```python
from build123d import *

# Parameters (mm, degrees)
F1_DEPTH = 50.8


with BuildPart() as f1:
    # F0 (on Front) → F1 (new body)
    with BuildSketch(Plane.XZ):
        with BuildLine():
            ThreePointArc((22.439383, 29.13105), (15.63549, 24.408793), (9.478033, 18.869985))
            Line((9.478033, 18.869985), (-23.461929, 58.559932))
            ThreePointArc((-23.461929, 58.559932), (-17.627724, 61.636811), (-12.409047, 57.603136))
            ThreePointArc((-12.409047, 57.603136), (-10.811238, 63.430969), (-12.409047, 69.258802))
            ThreePointArc((-12.409047, 69.258802), (-15.886595, 72.352499), (-20.328924, 73.741749))
            ThreePointArc((-20.328924, 73.741749), (-25.439806, 72.849507), (-30.041976, 70.454255))
            ThreePointArc((-30.041976, 70.454255), (-35.3729, 73.298377), (-41.398779, 73.741749))
            ThreePointArc((-41.398779, 73.741749), (-46.195621, 71.631394), (-49.169224, 67.316189))
            ThreePointArc((-49.169224, 67.316189), (-49.483254, 62.267433), (-47.525477, 57.603136))
            ThreePointArc((-47.525477, 57.603136), (-42.391887, 61.189751), (-37.258297, 57.603136))
            Line((-37.258297, 57.603136), (-37.258297, 32.199763))
            ThreePointArc((-37.258297, 32.199763), (-42.167966, 30.518016), (-46.330024, 27.41795))
            ThreePointArc((-46.330024, 27.41795), (-50.063504, 20.954714), (-50.81061, 13.528131))
            ThreePointArc((-50.81061, 13.528131), (-46.942892, 6.36599), (-39.005515, 4.562234))
            ThreePointArc((-39.005515, 4.562234), (-41.07612, 11.736213), (-37.258297, 18.153191))
            Line((-37.258297, 18.153191), (-37.258297, -18.857189))
            ThreePointArc((-37.258297, -18.857189), (-39.487397, -20.916304), (-42.500529, -21.276681))
            ThreePointArc((-42.500529, -21.276681), (-45.274392, -20.531283), (-47.608346, -18.857189))
            ThreePointArc((-47.608346, -18.857189), (-49.230344, -21.155103), (-49.355764, -23.965007))
            ThreePointArc((-49.355764, -23.965007), (-48.428049, -27.320039), (-46.398599, -30.148152))
            ThreePointArc((-46.398599, -30.148152), (-42.216094, -32.810312), (-37.258297, -32.836478))
            ThreePointArc((-37.258297, -32.836478), (-33.318107, -32.162609), (-29.865403, -30.148152))
            ThreePointArc((-29.865403, -30.148152), (-27.712308, -31.840895), (-25.160836, -32.836478))
            ThreePointArc((-25.160836, -32.836478), (-20.455986, -33.443738), (-16.020531, -31.761147))
            ThreePointArc((-16.020531, -31.761147), (-12.932619, -29.265174), (-10.912713, -25.846833))
            ThreePointArc((-10.912713, -25.846833), (-11.2086, -21.67018), (-13.063374, -17.916275))
            ThreePointArc((-13.063374, -17.916275), (-18.372816, -21.371176), (-23.682257, -17.916275))
            Line((-23.682257, -17.916275), (-23.682257, 15.553372))
            ThreePointArc((-23.682257, 15.553372), (-12.957597, 4.154356), (-6.669553, -10.177998))
            Line((-6.669553, -10.177998), (-6.669553, -54.607033))
            ThreePointArc((-6.669553, -54.607033), (-8.287699, -58.119332), (-11.300034, -60.544301))
            ThreePointArc((-11.300034, -60.544301), (-14.772838, -61.47915), (-17.679371, -59.361041))
            ThreePointArc((-17.679371, -59.361041), (-19.114876, -61.809201), (-19.297592, -64.641298))
            ThreePointArc((-19.297592, -64.641298), (-18.536614, -67.512258), (-16.814196, -69.931922))
            ThreePointArc((-16.814196, -69.931922), (-13.12521, -72.407987), (-8.715694, -72.95177))
            ThreePointArc((-8.715694, -72.95177), (-4.221828, -71.834414), (0, -69.931922))
            ThreePointArc((0, -69.931922), (4.559252, -71.907947), (9.41743, -72.95177))
            ThreePointArc((9.41743, -72.95177), (14.035159, -71.901137), (17.746311, -68.959267))
            ThreePointArc((17.746311, -68.959267), (19.072395, -63.743091), (17.746311, -58.526916))
            ThreePointArc((17.746311, -58.526916), (12.125868, -60.902929), (7.176861, -57.333316))
            ThreePointArc((7.176861, -57.333316), (6.708307, -55.925452), (6.564894, -54.448612))
            Line((6.564894, -54.448612), (7.254593, -9.766534))
            ThreePointArc((7.254593, -9.766534), (7.915044, -5.648664), (9.714889, -1.886536))
            Line((9.714889, -1.886536), (22.694213, -18.315103))
            ThreePointArc((22.694213, -18.315103), (17.190391, -21.190166), (11.686569, -18.315103))
            ThreePointArc((11.686569, -18.315103), (10.214197, -22.212635), (10.536366, -26.36653))
            ThreePointArc((10.536366, -26.36653), (13.072681, -30.734713), (17.444285, -33.265127))
            ThreePointArc((17.444285, -33.265127), (23.869566, -32.903906), (29.75891, -30.309618))
            ThreePointArc((29.75891, -30.309618), (35.644058, -32.921994), (42.081258, -32.773871))
            ThreePointArc((42.081258, -32.773871), (45.511296, -30.776469), (47.995683, -27.680892))
            ThreePointArc((47.995683, -27.680892), (48.784561, -22.594925), (46.756167, -17.864702))
            ThreePointArc((46.756167, -17.864702), (41.584109, -21.216198), (36.41205, -17.864702))
            Line((36.41205, -17.864702), (36.41205, 18.417337))
            ThreePointArc((36.41205, 18.417337), (41.00077, 11.851308), (39.371705, 4.008144))
            ThreePointArc((39.371705, 4.008144), (44.606315, 5.931777), (48.501298, 9.923093))
            ThreePointArc((48.501298, 9.923093), (50.482427, 16.674256), (48.501298, 23.425419))
            ThreePointArc((48.501298, 23.425419), (43.576958, 29.192803), (36.828664, 32.652915))
            Line((36.828664, 32.652915), (36.828664, 58.368564))
            ThreePointArc((36.828664, 58.368564), (41.780885, 61.482849), (46.733106, 58.368564))
            ThreePointArc((46.733106, 58.368564), (47.54337, 67.461962), (40.576808, 73.362254))
            ThreePointArc((40.576808, 73.362254), (34.734779, 72.917336), (29.45341, 70.380725))
            ThreePointArc((29.45341, 70.380725), (24.129346, 72.98331), (18.215336, 73.362254))
            ThreePointArc((18.215336, 73.362254), (11.281464, 67.4316), (12.336258, 58.368564))
            ThreePointArc((12.336258, 58.368564), (17.676832, 61.210114), (22.439383, 57.479933))
            Line((22.439383, 57.479933), (22.439383, 29.13105))
        make_face()
        with BuildLine():
            Line((-23.548043, 29.330348), (-23.548043, 39.393221))
            Line((-23.548043, 39.393221), (2.61824, 7.316703))
            Line((2.61824, 7.316703), (0, 1.270827))
            ThreePointArc((0, 1.270827), (-9.020803, 17.611136), (-23.548043, 29.330348))
        make_face(mode=Mode.SUBTRACT)
        with BuildLine():
            ThreePointArc((16.760936, 9.333754), (19.47767, 12.721904), (22.865819, 15.43864))
            Line((22.865819, 15.43864), (22.865819, 1.898702))
            Line((22.865819, 1.898702), (16.760936, 9.333754))
        make_face(mode=Mode.SUBTRACT)
    extrude(amount=F1_DEPTH)


solid = f1.part
```
CAD build for the part. Positions are in the model's coordinates, mm. A direction names the side the tool comes from. Coordinates: 2 decimals unless noted, no trailing zeros. Write each loop counter-clockwise with the first axis right and the second up, starting at its lowest first coordinate (ties: lowest second). Pieces come first, ordered by that corner, then holes. Notation, with made-up numbers: (-34.5, 6.5) -> (-8.5, 6.5) arc R14 cw to (-8.5, 10.5) -> close; hole circle Ø7 at (64, 64). An arc over 180 degrees is marked (long way). Use CSV: the item, a comma, the result in double quotes. Start each with the question number.
Item 1: Band-saw the part on D-D, the plane x = 25.5. Write the cut outline in (y, z), plus the area to 3 significant figures.
Item 2: Wall check: probe 1 along Z at (x, y) = (44, -37.5); probe 2 along Z at (x, y) = (38, -16.5); probe 3 along X at (y, z) = (-34.5, -2). Give the ranges that are in metal, low to high.
Item 3: Two-plate mould, pull along Z, no slides. Class faces 5 (the cylindrical face through (13.02, -25.04, -30.68)), 6 (the cylindrical face through (45.47, -25.04, -30.81)), 7 (the flat face through (-1, 0, 18)), 8 (the cylindrical face through (24.21, -25.04, 72.96)): +Z half, -Z half, draft (parallel to the pull), parting line (faces both ways), or undercut.
Item 4: Band-saw the part on A-A, the plane z = 42. Write the cut outline in (x, y).
Item 5: Drop flat-ended pins along their axis: P1, Ø22, axis at y = -14, z = -33.5, coming from the -X side; P2, Ø13, axis at y = -20, z = 46.5, coming from the +X side; P3, Ø2, axis at x = 40, y = -18, coming from the -Z side. Give the stop position or say it passes through.
Item 6: Band-saw the part on B-B, the plane z = -4. Write the cut outline in (x, y).
Item 7: Band-saw the part on C-C, the plane y = -18. Give the number of separate pieces and of enclosed holes in the cut face, plus the area to 3 significant figures.
Item 8: Tool access for faces 1 (the cylindrical face through (-49.22, -25.04, -21.12)), 2 (the cylindrical face through (-4.283, -25.044, -71.856)), 3 (the cylindrical face through (41.675, -25.044, -21.215)), 4 (the flat face through (36.829, -25, 45)): list every direction of +Z, -Z, +X, -X, +Y, -Y with a clear straight run to the whole face (end or side of a thin tool).
Response values:
1,outline,"(-50.8, -32.43) -> (0, -32.43) -> (0, 72.55) -> (-50.8, 72.55) -> close"
1,area,"5,330 mm2"
2,probe 1,"z = -31.87 to -20.68, 5.56 to 28.85, 61.01 to 71.86"
2,probe 2,"z = -33.2 to -19.94, 17.2 to 32.28, 59.98 to 73.44"
2,probe 3,"x = -37.26 to -23.68, -9.53 to 9.64, 9.8 to 36.41"
3,face 5,"undercut"
3,face 6,"-Z half"
3,face 7,"draft"
3,face 8,"+Z half"
4,outline,"(-37.26, -50.8) -> (-9.72, -50.8) -> (-9.72, 0) -> (-37.26, 0) -> close; (22.44, -50.8) -> (36.83, -50.8) -> (36.83, 0) -> (22.44, 0) -> close"
5,P1,"stops at x = -49.5"
5,P2,"stops at x = 36.83"
5,P3,"stops at z = -33.2"
6,outline,"(-37.26, -50.8) -> (-23.68, -50.8) -> (-23.68, 0) -> (-37.26, 0) -> close; (-8.67, -50.8) -> (8.54, -50.8) -> (8.54, 0) -> (-8.67, 0) -> close; (11.38, -50.8) -> (36.41, -50.8) -> (36.41, 0) -> (11.38, 0) -> close"
7,separate pieces,"1"
7,enclosed holes,"2"
7,area,"7,230 mm2"
8,face 1,"-X, +Y, -Y"
8,face 2,"-Z, +Y, -Y"
8,face 3,"+Y, -Y"
8,face 4,"+X, +Y, -Y"
